Input: part model. Units: mm. Frame: model coordinates. Round coordinates to 2 decimals unless told otherwise and drop trailing zeros. Loops run counter-clockwise (first coordinate to the right, second up) from the corner with the lowest first, then second, coordinate; pieces in that order, holes last. Notation, with made-up numbers: (46.25, -4) - (75.25, -4) arc R26 ccw to (75.25, 24) - close; hole circle Ø5 at (-9, 10.5). An arc over 180 degrees is marked (long way). One line per question, with ' | ' between items. Start each with the question number.
from build123d import *

# Parameters (mm, degrees)
F1_DEPTH = 25.4


# Not quite as in the source:
# - a feature names something its author has since deleted; it is built from what else it names


with BuildPart() as f1:
    # F0 (on Right) → F1 (new body)
    with BuildSketch(Plane.YZ):
        with BuildLine():
            ThreePointArc((41.1120694713, 5.3459768429), (37.5914213785, 3.215997322), (34.925, 6.35))
            Line((34.925, 6.35), (3.175, 6.35))
            Line((3.175, 6.35), (-3.175, 6.35))
            Line((-3.175, 6.35), (-29.7688, 6.35))
            ThreePointArc((-29.7688, 6.35), (-38.1, -1.9812), (-46.4312, 6.35))
            Line((-46.4312, 6.35), (-76.2, -6.35))
            Line((-76.2, -6.35), (-3.175, -6.35))
            Line((-3.175, -6.35), (-3.175, -4.7625))
            Line((-3.175, -4.7625), (0, -4.7625))
            Line((0, -4.7625), (3.175, -4.7625))
            Line((3.175, -4.7625), (3.175, -6.35))
            Line((3.175, -6.35), (76.2, -6.35))
            Line((76.2, -6.35), (41.1120694713, 5.3459768429))
        make_face()
    extrude(amount=F1_DEPTH)


solid = f1.part
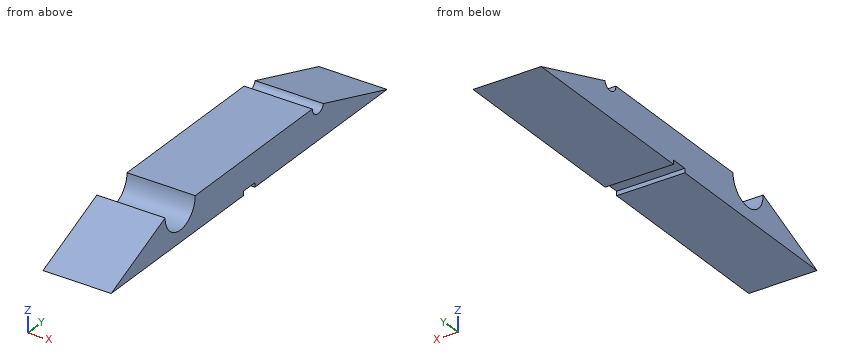
(1) Line query: line 1 along Z through (x, y) = (23.25, -43.5); line 2 along Z through (x, y) = (6, 54). Output: solid intervals per line, ascending. Write a range as from..to.
(2) Pin query (flat end, axial travel): P1, Ø6, axis at x = 7.5, z = 5, coming from the -Y side; P2, Ø1.9, axis at x = 17, y = 0.5, coming from the -Z side; P3, Ø1.3, axis at x = 8, z = -5.5, coming from the -Y side. Return the tip coordinate at first contact, or that it passes through.
(3) Section C-C, the plane y = -38.1. Output: boundary loops of the cut face in (x, z).
(4) Section D-D, the plane y = -54.5. Output: boundary loops of the cut face in (x, z), plus the area to 3 significant figures.
(5) Section A-A, the plane z = 0.75. Output: boundary loops of the cut face in (x, y), plus the area to 3 significant figures.
Derived:
1) line 1: z = -6.35..0.01 | line 2: z = -6.35..1.05
2) P1: stops at y = -56.63 | P2: stops at z = -4.76 | P3: stops at y = -75.73
3) outline: (0, -6.35) - (25.4, -6.35) - (25.4, -1.98) - (0, -1.98) - close
4) outline: (0, -6.35) - (25.4, -6.35) - (25.4, 2.91) - (0, 2.91) - close | area: 235 mm²
5) outline: (0, -59.56) - (25.4, -59.56) - (25.4, -44.27) - (0, -44.27) - close; (0, -31.93) - (25.4, -31.93) - (25.4, 54.9) - (0, 54.9) - close | area: 2,590 mm²
